The figure shows three views and two pictorial views of one solid part (mm, origin at its lowest corner). Answer the questions. Round coordinates to 2 decimals unless told otherwise and drop trailing zeros. Write each loop counter-clockwise with the first axis right and the second up, starting at its lowest first coordinate (ties: lowest second). Pieces come first, ordered by that corner, then holes.
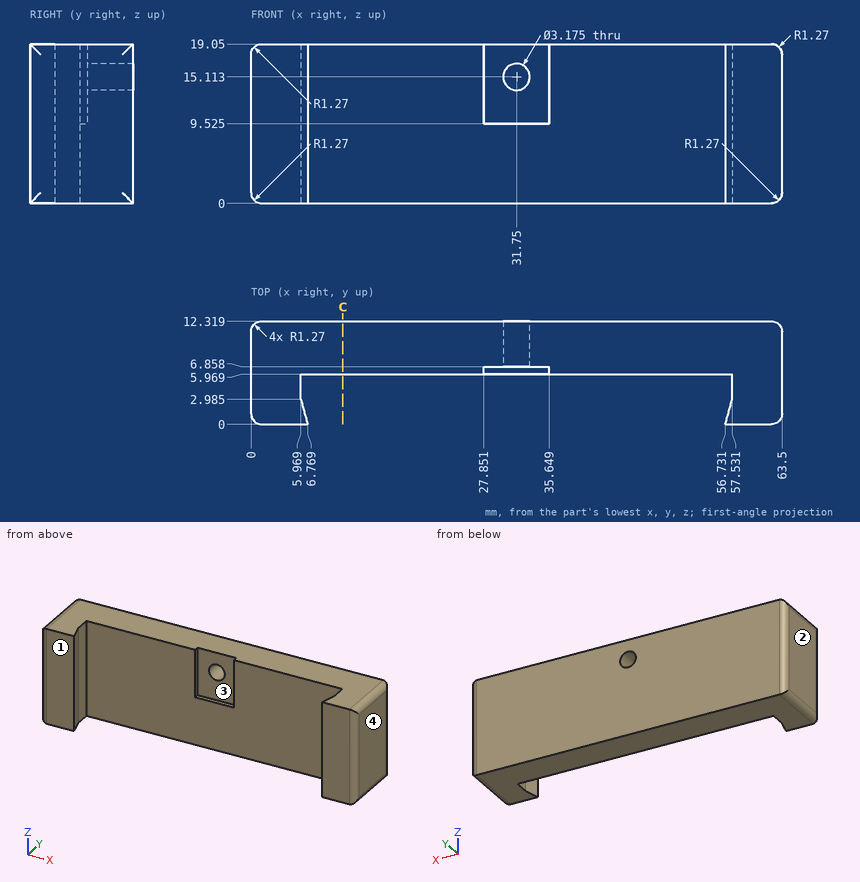
Q1. Section C-C (x = 11) is taken. Determine the outline of the cut face in (y, z), then the cut area to 3 significant figures.
Verdict:
outline: (5.97, 0) - (12.32, 0) - (12.32, 19.05) - (5.97, 19.05) - close
area: 121 mm2
Q2. Straight lines are drawn through the part: probe 1 along X at (y, z) = (4.75, 3.5); probe 2 along X at (y, z) = (6.25, 17.5); probe 3 along Y at (x, z) = (29.5, 16). For each, find the intervals that lie inside material, in ascending order.
Verdict:
probe 1: x = 0 to 5.97, 57.53 to 63.5
probe 2: x = 0 to 27.85, 35.65 to 63.5
probe 3: y = 6.86 to 12.32
Q3. Determine the mould class of the marked faces 1, 2, 3 and 4 for opening direction X: pulls with the +X half, pulls with the -X half, needs draft (parallel to the pull), parting line crosses it, or undercut.
Verdict:
face 1: needs draft
face 2: pulls with the -X half
face 3: undercut
face 4: pulls with the +X half
Q4. A flat-ended cylindrical pin translates along its axis: pin 1 Ø1 at (x, z) = (32, 11.5) entering from -Y. Find the tip coordinate at first contact, or state that the pin passes through.
Verdict:
pin 1: stops at y = 6.86
